Here's how the part is built. I have some questions about the finished solid (model axes, mm). A direction names the side the tool comes from. Round coordinates to 2 decimals unless told otherwise and drop trailing zeros. Loops run counter-clockwise (first coordinate to the right, second up) from the corner with the lowest first, then second, coordinate; pieces in that order, holes last. Notation, with made-up numbers: M -31.75,45 L -17.75,45 A13 ccw -17.75,49 Z; hole C -8,69.25 d2. An arc over 180 degrees is marked long. One line per question, with ' | ' between items. Start each with the question number.
```python
from build123d import *

# Parameters (mm, degrees)
SKETCH1_W                                           = 120
SKETCH1_H                                           = 90
SKETCH1_R                                           = 41.25
BOSS_EXTRUDE1_DEPTH                                 = 3
SKETCH2_W                                           = 120
SKETCH2_H                                           = 90
BOSS_EXTRUDE2_DEPTH                                 = 8
CBORE_FOR_M4_HEX_SOCKET_HEAD_CAP_SCREW1_D           = 4.8
CBORE_FOR_M4_HEX_SOCKET_HEAD_CAP_SCREW1_CBORE_D     = 8
CBORE_FOR_M4_HEX_SOCKET_HEAD_CAP_SCREW1_CBORE_DEPTH = 4.4
SKETCH5_W                                           = 20
SKETCH5_H                                           = 90
BOSS_EXTRUDE3_DEPTH                                 = 90
SKETCH8_R                                           = 32
CUT_EXTRUDE3_DEPTH                                  = 150.083869013
M5_CLEARANCE_HOLE1_D                                = 5.8
CUT_EXTRUDE4_START                                  = -8
SKETCH13_R                                          = 43
SKETCH13_R_2                                        = 6.9
SKETCH13_R_3                                        = 2.9
SKETCH13_R_4                                        = 32
CUT_EXTRUDE4_DEPTH                                  = 8
FILLET1_R                                           = 8
SKETCH14_W                                          = 17
SKETCH14_H                                          = 90
BOSS_EXTRUDE4_DEPTH                                 = 70
TAP_DRILL_FOR_M3_TAP2_D                             = 2.5
CUT_EXTRUDE5_DEPTH                                  = 152.112541008
SKETCH21_W                                          = 81
SKETCH21_H                                          = 90
CUT_EXTRUDE6_DEPTH                                  = 13
BOSS_EXTRUDE5_DEPTH                                 = 10
BOSS_EXTRUDE6_START                                 = -90
BOSS_EXTRUDE6_DEPTH                                 = 10
FILLET3_R                                           = 5
FILLET2_R                                           = 20
FILLET4_R                                           = 10


with BuildPart() as part:
    # Sketch1 → Boss-Extrude1 (new body)
    with BuildSketch(Plane.XY):
        Rectangle(SKETCH1_W, SKETCH1_H)
        Circle(SKETCH1_R, mode=Mode.SUBTRACT)
    extrude(amount=BOSS_EXTRUDE1_DEPTH)

    # Sketch2 → Boss-Extrude2 (add)
    with BuildSketch(Plane.XY.offset(3)):
        Rectangle(SKETCH2_W, SKETCH2_H)
    extrude(amount=BOSS_EXTRUDE2_DEPTH)

    # CBORE for M4 Hex Socket Head Cap Screw1 (through all)
    with Locations(Plane.XY.offset(11)):
        with Locations((-21.25, 0), (0, 21.25), (21.25, 0), (0, -21.25)):
            CounterBoreHole(CBORE_FOR_M4_HEX_SOCKET_HEAD_CAP_SCREW1_D / 2, CBORE_FOR_M4_HEX_SOCKET_HEAD_CAP_SCREW1_CBORE_D / 2, CBORE_FOR_M4_HEX_SOCKET_HEAD_CAP_SCREW1_CBORE_DEPTH)

    # Sketch5 → Boss-Extrude3 (add)
    with BuildSketch(Plane.XY.offset(11)):
        with Locations((50, 0)):
            Rectangle(SKETCH5_W, SKETCH5_H)
    extrude(amount=BOSS_EXTRUDE3_DEPTH)

    # Sketch8 → Cut-Extrude3 (cut, through all)
    with BuildSketch(Plane.ZY.offset(-40)):
        with Locations(Location((56, 0, 0), (0, 0, 270))):
            Circle(SKETCH8_R)
    extrude(amount=-CUT_EXTRUDE3_DEPTH, mode=Mode.SUBTRACT)

    # M5 Clearance Hole1 (through all)
    with Locations(Plane(origin=(60, 0, 0), x_dir=(0, 0, -1), z_dir=(1, 0, 0))):
        with Locations((-22.412427894, -33.587572106), (-89.587572106, -33.587572106), (-89.587572106, 33.587572106), (-22.412427894, 33.587572106)):
            Hole(M5_CLEARANCE_HOLE1_D / 2)

    # Sketch13 → Cut-Extrude4 (cut)
    # profile 1 of 22: a face of its own
    with BuildSketch(Plane(origin=(60, 0, 0), x_dir=(0, 0, -1), z_dir=(1, 0, 0)).offset(CUT_EXTRUDE4_START)):
        with Locations((-56, 0)):
            Circle(SKETCH13_R)
    # profile 2 of 22: a face of its own
    with BuildSketch(Plane(origin=(60, 0, 0), x_dir=(0, 0, -1), z_dir=(1, 0, 0)).offset(CUT_EXTRUDE4_START)):
        with Locations((-89.587572106, 33.587572106)):
            Circle(SKETCH13_R_2)
        with Locations((-89.587572106, 33.587572106)):
            Circle(SKETCH13_R_3, mode=Mode.SUBTRACT)
    # profile 3 of 22: a face of its own
    with BuildSketch(Plane(origin=(60, 0, 0), x_dir=(0, 0, -1), z_dir=(1, 0, 0)).offset(CUT_EXTRUDE4_START)):
        with Locations((-56, 0)):
            Circle(SKETCH13_R)
    # profile 4 of 22: a face of its own
    with BuildSketch(Plane(origin=(60, 0, 0), x_dir=(0, 0, -1), z_dir=(1, 0, 0)).offset(CUT_EXTRUDE4_START)):
        with Locations((-89.587572106, 33.587572106)):
            Circle(SKETCH13_R_2)
    # profile 5 of 22: a face of its own
    with BuildSketch(Plane(origin=(60, 0, 0), x_dir=(0, 0, -1), z_dir=(1, 0, 0)).offset(CUT_EXTRUDE4_START)):
        with Locations((-22.412427894, 33.587572106)):
            Circle(SKETCH13_R_2)
    # profile 6 of 22: a face of its own
    with BuildSketch(Plane(origin=(60, 0, 0), x_dir=(0, 0, -1), z_dir=(1, 0, 0)).offset(CUT_EXTRUDE4_START)):
        with Locations((-56, 0)):
            Circle(SKETCH13_R)
        with Locations(Location((-56, 0, 0), (0, 0, 270))):
            Circle(SKETCH13_R_4, mode=Mode.SUBTRACT)
    # profile 7 of 22: a face of its own
    with BuildSketch(Plane(origin=(60, 0, 0), x_dir=(0, 0, -1), z_dir=(1, 0, 0)).offset(CUT_EXTRUDE4_START)):
        with Locations((-89.587572106, 33.587572106)):
            Circle(SKETCH13_R_2)
    # profile 8 of 22: a face of its own
    with BuildSketch(Plane(origin=(60, 0, 0), x_dir=(0, 0, -1), z_dir=(1, 0, 0)).offset(CUT_EXTRUDE4_START)):
        with Locations((-89.587572106, -33.587572106)):
            Circle(SKETCH13_R_2)
    # profile 9 of 22: a face of its own
    with BuildSketch(Plane(origin=(60, 0, 0), x_dir=(0, 0, -1), z_dir=(1, 0, 0)).offset(CUT_EXTRUDE4_START)):
        with Locations((-22.412427894, -33.587572106)):
            Circle(SKETCH13_R_2)
    # profile 10 of 22: a face of its own
    with BuildSketch(Plane(origin=(60, 0, 0), x_dir=(0, 0, -1), z_dir=(1, 0, 0)).offset(CUT_EXTRUDE4_START)):
        with Locations((-56, 0)):
            Circle(SKETCH13_R)
    # profile 11 of 22: a face of its own
    with BuildSketch(Plane(origin=(60, 0, 0), x_dir=(0, 0, -1), z_dir=(1, 0, 0)).offset(CUT_EXTRUDE4_START)):
        with Locations((-22.412427894, 33.587572106)):
            Circle(SKETCH13_R_2)
    # profile 12 of 22: a face of its own
    with BuildSketch(Plane(origin=(60, 0, 0), x_dir=(0, 0, -1), z_dir=(1, 0, 0)).offset(CUT_EXTRUDE4_START)):
        with Locations((-56, 0)):
            Circle(SKETCH13_R)
    # profile 13 of 22: a face of its own
    with BuildSketch(Plane(origin=(60, 0, 0), x_dir=(0, 0, -1), z_dir=(1, 0, 0)).offset(CUT_EXTRUDE4_START)):
        with Locations((-22.412427894, 33.587572106)):
            Circle(SKETCH13_R_2)
        with Locations((-22.412427894, 33.587572106)):
            Circle(SKETCH13_R_3, mode=Mode.SUBTRACT)
    # profile 14 of 22: a face of its own
    with BuildSketch(Plane(origin=(60, 0, 0), x_dir=(0, 0, -1), z_dir=(1, 0, 0)).offset(CUT_EXTRUDE4_START)):
        with Locations((-56, 0)):
            Circle(SKETCH13_R)
    # profile 15 of 22: a face of its own
    with BuildSketch(Plane(origin=(60, 0, 0), x_dir=(0, 0, -1), z_dir=(1, 0, 0)).offset(CUT_EXTRUDE4_START)):
        with Locations((-22.412427894, -33.587572106)):
            Circle(SKETCH13_R_2)
    # profile 16 of 22: a face of its own
    with BuildSketch(Plane(origin=(60, 0, 0), x_dir=(0, 0, -1), z_dir=(1, 0, 0)).offset(CUT_EXTRUDE4_START)):
        with Locations((-56, 0)):
            Circle(SKETCH13_R)
    # profile 17 of 22: a face of its own
    with BuildSketch(Plane(origin=(60, 0, 0), x_dir=(0, 0, -1), z_dir=(1, 0, 0)).offset(CUT_EXTRUDE4_START)):
        with Locations((-22.412427894, -33.587572106)):
            Circle(SKETCH13_R_2)
        with Locations((-22.412427894, -33.587572106)):
            Circle(SKETCH13_R_3, mode=Mode.SUBTRACT)
    # profile 18 of 22: a face of its own
    with BuildSketch(Plane(origin=(60, 0, 0), x_dir=(0, 0, -1), z_dir=(1, 0, 0)).offset(CUT_EXTRUDE4_START)):
        with Locations((-56, 0)):
            Circle(SKETCH13_R)
    # profile 19 of 22: a face of its own
    with BuildSketch(Plane(origin=(60, 0, 0), x_dir=(0, 0, -1), z_dir=(1, 0, 0)).offset(CUT_EXTRUDE4_START)):
        with Locations((-89.587572106, -33.587572106)):
            Circle(SKETCH13_R_2)
    # profile 20 of 22: a face of its own
    with BuildSketch(Plane(origin=(60, 0, 0), x_dir=(0, 0, -1), z_dir=(1, 0, 0)).offset(CUT_EXTRUDE4_START)):
        with Locations((-56, 0)):
            Circle(SKETCH13_R)
    # profile 21 of 22: a face of its own
    with BuildSketch(Plane(origin=(60, 0, 0), x_dir=(0, 0, -1), z_dir=(1, 0, 0)).offset(CUT_EXTRUDE4_START)):
        with Locations((-89.587572106, -33.587572106)):
            Circle(SKETCH13_R_2)
        with Locations((-89.587572106, -33.587572106)):
            Circle(SKETCH13_R_3, mode=Mode.SUBTRACT)
    # profile 22 of 22: a face of its own
    with BuildSketch(Plane(origin=(60, 0, 0), x_dir=(0, 0, -1), z_dir=(1, 0, 0)).offset(CUT_EXTRUDE4_START)):
        with Locations((-22.412427894, -33.587572106)):
            Circle(SKETCH13_R_3)
    extrude(amount=CUT_EXTRUDE4_DEPTH, mode=Mode.SUBTRACT)

    # Fillet1
    fillet1_edges = [part.edges().sort_by_distance(p)[0] for p in [
        (56, 26.688751419, 89.715138257),
        (56, 33.715138257, 82.688751419),
        (56, 33.715138257, 29.311248581),
        (56, 26.688751419, 22.284861743),
        (56, -26.688751419, 22.284861743),
        (56, -33.715138257, 29.311248581),
        (56, -33.715138257, 82.688751419),
        (56, -26.688751419, 89.715138257),
    ]]
    fillet(fillet1_edges, radius=FILLET1_R)

    # Sketch14 → Boss-Extrude4 (add)
    with BuildSketch(Plane.XY.offset(11)):
        with Locations((-51.5, 0)):
            Rectangle(SKETCH14_W, SKETCH14_H)
    extrude(amount=BOSS_EXTRUDE4_DEPTH)

    # Tap Drill for M3 Tap2 (through all)
    with Locations(Plane(origin=(-43, 0, 0), x_dir=(0, 0, -1), z_dir=(1, 0, 0))):
        with Locations((-71, -24), (-71, 24), (-41, -24), (-41, 24)):
            Hole(TAP_DRILL_FOR_M3_TAP2_D / 2)

    # Sketch20 → Cut-Extrude5 (cut, through all)
    with BuildSketch(Plane(origin=(-43, 0, 0), x_dir=(0, 0, -1), z_dir=(1, 0, 0))):
        with BuildLine():
            ThreePointArc((-66.75, 24), (-67.99479618, 20.99479618), (-71, 19.75))
            Line((-71, 19.75), (-71, -19.75))
            ThreePointArc((-71, -19.75), (-67.99479618, -20.99479618), (-66.75, -24))
            Line((-66.75, -24), (-45.25, -24))
            ThreePointArc((-45.25, -24), (-44.00520382, -20.99479618), (-41, -19.75))
            Line((-41, -19.75), (-41, 19.75))
            ThreePointArc((-41, 19.75), (-44.00520382, 20.99479618), (-45.25, 24))
            Line((-45.25, 24), (-66.75, 24))
        make_face()
    extrude(amount=-CUT_EXTRUDE5_DEPTH, mode=Mode.SUBTRACT)

    # Sketch21 → Cut-Extrude6 (cut)
    with BuildSketch(Plane.ZY.offset(60)):
        with Locations((40.5, 0)):
            Rectangle(SKETCH21_W, SKETCH21_H)
    extrude(amount=-CUT_EXTRUDE6_DEPTH, mode=Mode.SUBTRACT)

    # Sketch22 → Boss-Extrude5 (add)
    with BuildSketch(Plane.XZ.offset(45)):
        Polygon((-43, 81), (-25, 11), (-43, 11), align=None)
    extrude(amount=-BOSS_EXTRUDE5_DEPTH)

    # Sketch22<2> → Boss-Extrude6 (add)
    with BuildSketch(Plane.XZ.offset(45).offset(BOSS_EXTRUDE6_START)):
        Polygon((-43, 81), (-25, 11), (-43, 11), align=None)
    extrude(amount=BOSS_EXTRUDE6_DEPTH)

    # Fillet3
    fillet3_edges = [part.edges().sort_by_distance(p)[0] for p in [
        (-43, -35, 46),
        (-43, 35, 46),
    ]]
    fillet(fillet3_edges, radius=FILLET3_R)

    # Fillet2
    # the kernel refuses this fillet: 20 mm, written as the material it takes off along each edge
    with BuildSketch(Plane(origin=(-97, 45, 81), x_dir=(0, -1, 0), z_dir=(1, 0, 0)), Plane(origin=(7, -45, 81), x_dir=(0, 1, 0), z_dir=(-1, 0, 0))) as fillet2_piece_1:
        with BuildLine():
            CenterArc((FILLET2_R, FILLET2_R), FILLET2_R, 180, 90)
            Line((0, FILLET2_R), (0, 0))
            Line((0, 0), (FILLET2_R, 0))
        make_face()
    extrude(amount=104, mode=Mode.SUBTRACT)

    # Fillet4
    fillet4_edges = [part.edges().sort_by_distance(p)[0] for p in [
        (50, 45, 101),
        (50, -45, 101),
    ]]
    fillet(fillet4_edges, radius=FILLET4_R)


solid = part.part
```
1) Imagine slicing it at D-D (x = 48). Write out the boundary of the cut face in (y, z), then the cut area to 3 significant figures.
2) Imagine slicing it at C-C (x = 28). Write out the boundary of the cut face in (y, z), then the cut area to 3 significant figures.
3) For faces 1 (the face through (56, 43, 56)), 2 (the face through (-0.521, 25.216, 8.831)), 3 (the face through (0.52, 18.907, 4.775)), which set-ups out of +Z, -Z, +X, -X, +Y, -Y let a thin tool reach every point of the face, with its end or its side?
4) We'd pull the mould along X, two halves only. Please class faces 4 (the face through (52, -19, 28)), 5 (the face through (-44.97, -21.03, 44.04)), 6 (the face through (0.52, -23.593, 4.775)): pulls with the +X half, pulls with the -X half, needs draft (parallel to the pull), parting line crosses it, or undercut.
5) Imagine slicing it at A-A (z = 56). Write out the boundary of the cut face in (x, y).
6) I'm going to push flat-ended pins straight in: pin 1 Ø9 at (x, y) = (21, 0.5) entering from +Z; pin 2 Ø9.5 at (y, z) = (33.59, 22.41) entering from +X; pin 3 Ø4.5 at (x, y) = (-45, 6) entering from +Z. Where does each tip first touch, or does it pass through?
7) Please list where these lines run through material, in increasing order: L1, parallel to Y at x = 0, z = 7.6; L2, parallel to Y at x = -21, z = 8; L3, parallel to X at y = 23, z = 20.5. Write a range as from..to.
8) Imagine slicing it at B-B (y = -10). Write out the boundary of the cut face in (x, z).
Results are:
1) outline: M -45,0 L 45,0 L 45,91 A10 ccw 35,101 L -35,101 A10 ccw -45,91 Z; hole C -33.59,22.41 d5.8; hole C -33.59,89.59 d5.8; hole C 0,56 d64; hole C 33.59,22.41 d5.8; hole C 33.59,89.59 d5.8 | area: 5,720 mm²
2) outline: M -45,0 L -30.29,0 L -30.29,3 L 30.29,3 L 30.29,0 L 45,0 L 45,11 L -45,11 Z | area: 808 mm²
3) face 1: +X | face 2: +Z | face 3: +Z, -Z
4) face 4: pulls with the +X half | face 5: needs draft | face 6: undercut
5) outline: M -47,-45 L -36.57,-45 L -36.57,-35 L -38,-35 A5 cw -43,-30 L -43,-24 L -47,-24 Z; M -47,24 L -43,24 L -43,30 A5 cw -38,35 L -36.57,35 L -36.57,45 L -47,45 Z; M 40,-45 L 60,-45 L 60,-43 L 52,-43 L 52,-32 L 40,-32 Z; M 40,32 L 52,32 L 52,43 L 60,43 L 60,45 L 40,45 Z
6) pin 1: z = 11 | pin 2: x = 52 | pin 3: z = 81
7) L1: -45..-25.25, -17.25..17.25, 25.25..45 | L2: -45..-3.99, 3.99..45 | L3: -47..-43, 40..52
8) outline: M -47,0 L -40.02,0 L -40.02,3 L 40.02,3 L 40.02,0 L 60,0 L 60,14.18 L 52,14.18 L 52,25.6 L 40,25.6 L 40,11 L -43,11 L -43,41 L -47,41 Z; M -47,71 L -43,71 L -43,81 L -47,81 Z; M 40,86.4 L 52,86.4 L 52,97.82 L 60,97.82 L 60,101 L 40,101 Z
